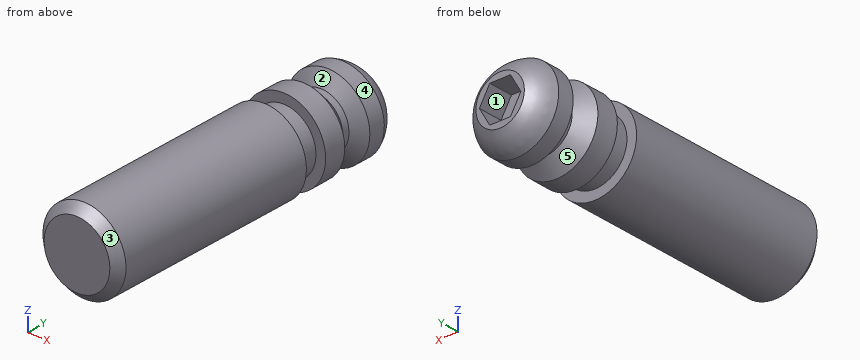
from build123d import *

# Parameters (mm, degrees)
SKETCH1_R           = 3
BOSS_EXTRUDE1_DEPTH = 23.5
CHAMFER1_SIZE       = 0.625
CUT_EXTRUDE1_DEPTH  = 1.8


with BuildPart() as part:
    # Sketch1 → Boss-Extrude1 (new body)
    with BuildSketch(Plane(origin=(0, 0, 0), x_dir=(1, 0, 0), z_dir=(0, 1, 0))):
        with Locations(Location((0, 0, 0), (0, 0, 270))):
            Circle(SKETCH1_R)
    extrude(amount=BOSS_EXTRUDE1_DEPTH)

    # Sketch2 → Cut-Revolve1 (revolve, cut)
    with BuildSketch(Plane.XY, mode=Mode.PRIVATE) as cut_revolve1_sk:
        with BuildLine():
            Line((3, 22.081556921), (3, 20.881556921))
            Line((3, 20.881556921), (1.995368836, 20.301532848))
            Line((1.995368836, 20.301532848), (1.995368836, 19.801532848))
            Line((1.995368836, 19.801532848), (2.986803407, 18.810098278))
            Line((2.986803407, 18.810098278), (3, 17.210098278))
            Line((3, 17.210098278), (2.3, 17.210098278))
            Line((2.3, 17.210098278), (2.3, 15.610098278))
            Line((2.3, 15.610098278), (3, 15.610098278))
            Line((3, 15.610098278), (5.142193945, 15.610098278))
            Line((5.142193945, 15.610098278), (5.142193945, 23.5))
            Line((5.142193945, 23.5), (1.75, 23.5))
            ThreePointArc((1.75, 23.5), (2.493968727, 22.895619403), (3, 22.081556921))
        make_face()
    revolve(cut_revolve1_sk.sketch.rotate(Axis((0, 23.5, 0), (0, -1, 0)), 90), axis=Axis((0, 23.5, 0), (0, -1, 0)), mode=Mode.SUBTRACT)

    # Chamfer1
    chamfer1_edges = [part.edges().sort_by_distance(p)[0] for p in [
        (0, 0, -3),
    ]]
    chamfer(chamfer1_edges, length=CHAMFER1_SIZE)

    # Sketch3 → Cut-Extrude1 (cut)
    with BuildSketch(Plane(origin=(0, 23.5, 0), x_dir=(1, 0, 0), z_dir=(0, 1, 0))):
        Polygon((0.745992991, -1.301343328), (1.499992877, -0.004622783), (0.753999886, 1.296720545), (-0.745992991, 1.301343328), (-1.499992877, 0.004622783), (-0.753999886, -1.296720545), align=None)
    extrude(amount=-CUT_EXTRUDE1_DEPTH, mode=Mode.SUBTRACT)


solid = part.part
For this review, take the finished solid that the model builds, in its own axes (mm). Face numbers are marked on the shaded views. A direction names the side the tool comes from. Round coordinates to 2 decimals unless told otherwise and drop trailing zeros. Write each loop counter-clockwise with the first axis right and the second up, starting at its lowest first coordinate (ties: lowest second). Pieces come first, ordered by that corner, then holes. Notation, with made-up numbers: (74.5, 26) - (93.5, 26) arc R29 cw to (93.5, 58) - close; hole circle Ø2 at (74, 56.25). An arc over 180 degrees is marked (long way). Use a Markdown table: item, result.
Q1. Machinability: for the marked faces 1, 2 and 3, which of the approach directions +Z, -Z, +X, -X, +Y, -Y give a long, thin tool a straight path to every point of the face, cutting with its end or side? Answer none if there is none.
Derived:
| item | result |
|---|---|
| face 1 | +Y |
| face 2 | none |
| face 3 | -Y |
Q2. Clearance check with flat-ended pins moving along their axes: pin 1 (1.8 mm diameter, centred on x = 0, z = 0, fed in from -Y); pin 2 (1 mm diameter, centred on y = 18.5, z = -1.5, fed in from -X); pin 3 (1 mm diameter, centred on y = 15.5, z = 2, fed in from +X); pin 4 (1 mm diameter, centred on y = 6.5, z = -2, fed in from -X). State where each tip first meets the part, or that it passes through.
Derived:
| item | result |
|---|---|
| pin 1 | stops at y = 0 |
| pin 2 | stops at x = -2.82 |
| pin 3 | stops at x = 2.6 |
| pin 4 | stops at x = -2.6 |
Q3. Wall thickness on line 1 along Y through (x, z) = (-0.75, -1); line 2 along Y through (x, z) = (2.25, 0.25); line 3 along Z through (x, y) = (-1, 21.75): over which ranges is each line inside the solid? List them lowest first.
Derived:
| item | result |
|---|---|
| line 1 | y = 0 to 21.7 |
| line 2 | y = 0 to 19.53, 20.46 to 23.13 |
| line 3 | z = -2.83 to -0.86, 0.87 to 2.83 |
Q4. We need section B-B (y = 6). Give the boundary of the cut face in (x, z).
Derived:
| item | result |
|---|---|
| outline | circle Ø6 at (0, 0) |
Q5. We need section A-A (z = 2.75). State how many separate pieces and enclosed holes the cut face has, plus the area to 3 significant figures.
Derived:
| item | result |
|---|---|
| separate pieces | 3 |
| enclosed holes | 0 |
| area | 44.4 mm2 |
Q6. The part is to be moulded in two halves that separate along Y. For the marked faces 4 and 5, say which applies: pulls with the +Y half, pulls with the -Y half, needs draft (parallel to the pull), parting line crosses it, or undercut.
Derived:
| item | result |
|---|---|
| face 4 | needs draft |
| face 5 | undercut |
